```python
from build123d import *

# Parameters (mm, degrees)
F0_W            = 101.6
F0_H            = 65.024
F0_R            = 9.525
F1_DEPTH        = 31.75
F3_DEPTH        = 101.601
F5_START        = -63.5
F5_DEPTH        = 38.1
F6_DEPTH        = 38.1
F7_R            = 4.7625
F8_DEPTH        = 15.875
F9_R            = 4.7625
F10_DEPTH       = 15.875
F12_D           = 9.525
F12_CBORE_D     = 12.7
F12_CBORE_DEPTH = 6.35


with BuildPart() as f1:
    # F0 (on Top) → F1 (new body)
    with BuildSketch(Plane.XY):
        Rectangle(F0_W, F0_H)
        Circle(F0_R, mode=Mode.SUBTRACT)
    extrude(amount=F1_DEPTH)

    # F2 (on face) → F3 (cut, through all)
    with BuildSketch(Plane.YZ.offset(50.8)):
        with BuildLine():
            Line((19.812, 6.35), (-19.812, 6.35))
            ThreePointArc((-19.812, 6.35), (-24.3021280605, 4.4901280605), (-26.162, 0))
            Line((-26.162, 0), (26.162, 0))
            ThreePointArc((26.162, 0), (24.3021280605, 4.4901280605), (19.812, 6.35))
        make_face()
    extrude(amount=-F3_DEPTH, mode=Mode.SUBTRACT)

    # F4 (on face) → F5 (join)
    with BuildSketch(Plane.YZ.offset(50.8).offset(F5_START)):
        Polygon((-18.288, 38.1), (-18.288, 31.75), (19.812, 31.75), (19.812, 38.1), (26.924, 38.1), (26.924, 69.85), (19.812, 69.85), (4.064, 54.102), (4.064, 47.752), (-2.54, 47.752), (-2.54, 54.102), (-18.288, 69.85), (-25.4, 69.85), (-25.4, 38.1), align=None)
    extrude(amount=-F5_DEPTH)

    # F4 (on face) → F6 (join)
    with BuildSketch(Plane.YZ.offset(50.8)):
        Polygon((-18.288, 38.1), (-18.288, 31.75), (19.812, 31.75), (19.812, 38.1), (26.924, 38.1), (26.924, 69.85), (19.812, 69.85), (4.064, 54.102), (4.064, 47.752), (-2.54, 47.752), (-2.54, 54.102), (-18.288, 69.85), (-25.4, 69.85), (-25.4, 38.1), align=None)
    extrude(amount=-F6_DEPTH)

    # F7 (on face) → F8 (cut)
    with BuildSketch(Plane.YZ.offset(50.8)):
        with Locations((0, 22.225)):
            Circle(F7_R)
    extrude(amount=-F8_DEPTH, mode=Mode.SUBTRACT)

    # F9 (on face) → F10 (cut)
    with BuildSketch(Plane(origin=(-50.8, 0, 0), x_dir=(0, -1, 0), z_dir=(-1, 0, 0))):
        with Locations((0, 22.225)):
            Circle(F9_R)
    extrude(amount=-F10_DEPTH, mode=Mode.SUBTRACT)

    # F12 (through all)
    with Locations(Plane.XZ.offset(32.512)):
        with Locations((0, 15.875)):
            CounterBoreHole(F12_D / 2, F12_CBORE_D / 2, F12_CBORE_DEPTH)


solid = f1.part
```
Part model, mm, in its own coordinate system. A direction names the side the tool comes from. Round coordinates to 2 decimals unless told otherwise and drop trailing zeros. Loops run counter-clockwise (first coordinate to the right, second up) from the corner with the lowest first, then second, coordinate; pieces in that order, holes last.
Item 1: Drill centre lines: line 1 (X direction, y = 26, z = 16); line 2 (Z direction, x = 41.5, y = 0); line 3 (X direction, y = -10.5, z = 34). Where is each one in solid material? Low to high.
Item 2: Cut at A-A, the plane x = 0. State how many separate pieces and enclosed holes the cut face has, then the cut area to 3 significant figures.
Item 3: Cut at D-D, the plane x = -20. Give the cut face in (y, z).
Item 4: Mould opens along Y. For faces 4 (the face through (42.974, -0.62, 26.947)), 5 (the face through (-31, -22, 38.1)), 6 (the face through (32, 26.924, 54)) say: +Y half, -Y half, draft (parallel to the pull), parting line (faces both ways), or undercut.
Item 5: Drop flat-ended pins along their axis: P1, Ø7, axis at x = 22.5, z = 50, coming from the +Y side; P2, Ø8, axis at x = 5.5, y = -11, coming from the -Z side; P3, Ø10.5, axis at y = 2, z = 20.5, coming from the +X side; P4, Ø7.5, axis at x = 23.5, y = 1, coming from the +Z side. Give the stop position or say it passes through.
Item 6: 3-axis set-ups, long thin cutter, end or side, ignore diameter. For faces 1 (the face through (1, -26.162, 21)), 2 (the face through (32, -18.288, 35)), 3 (the face through (32.02, 12.05, 62.09)): which of +Z, -Z, +X, -X, +Y, -Y reach the whole face in a straight line?
Item 7: Cut at C-C, the plane z = 49. Give the cut face in (x, y).
A:
1. line 1: x = -50.8 to -4.76, 4.76 to 50.8
1. line 2: z = 6.35 to 17.46, 26.99 to 47.75
1. line 3: x = -50.8 to -12.7, 12.7 to 50.8
2. separate pieces: 4
2. enclosed holes: 0
2. area: 808 mm2
3. outline: (-32.51, 0) - (-26.16, 0) arc R6.35 cw to (-19.81, 6.35) - (19.81, 6.35) arc R6.35 cw to (26.16, 0) - (32.51, 0) - (32.51, 31.75) - (19.81, 31.75) - (19.81, 38.1) - (26.92, 38.1) - (26.92, 69.85) - (19.81, 69.85) - (4.06, 54.1) - (4.06, 47.75) - (-2.54, 47.75) - (-2.54, 54.1) - (-18.29, 69.85) - (-25.4, 69.85) - (-25.4, 38.1) - (-18.29, 38.1) - (-18.29, 31.75) - (-32.51, 31.75) - close
4. face 4: undercut
4. face 5: draft
4. face 6: +Y half
5. P1: stops at y = 26.92
5. P2: stops at z = 6.35
5. P3: stops at x = 50.8
5. P4: stops at z = 54.79
6. face 1: -Y
6. face 2: +X, -X, -Y
6. face 3: +Z, +X, -X
7. outline: (-50.8, -25.4) - (-12.7, -25.4) - (-12.7, -2.54) - (-50.8, -2.54) - close; (-50.8, 4.06) - (-12.7, 4.06) - (-12.7, 26.92) - (-50.8, 26.92) - close; (12.7, -25.4) - (50.8, -25.4) - (50.8, -2.54) - (12.7, -2.54) - close; (12.7, 4.06) - (50.8, 4.06) - (50.8, 26.92) - (12.7, 26.92) - close
